Input: part model. Units: mm. Frame: model coordinates. Face numbers are marked on the shaded views. A direction names the side the tool comes from. Give positions to 0.01 mm unless a question says otherwise; leave off trailing zeros. Loops run counter-clockwise (first coordinate to the right, second up) from the corner with the lowest first, then second, coordinate; pieces in that order, holes last. Notation, with made-up numbers: (-17.75, 8.5) -> (-9.75, 8.5) arc R28 ccw to (-9.75, 29.5) -> close; hole circle Ø11 at (3, -28). An arc over 180 degrees is marked (long way). One line per question, with ' | ' between items.
from build123d import *

# Parameters (mm, degrees)
SKETCH1_W           = 120
SKETCH1_H           = 70
BOSS_EXTRUDE1_DEPTH = 10
SKETCH1_3_W         = 20
SKETCH1_3_H         = 70
SKETCH1_3_H_2       = 5.314701235
BOSS_EXTRUDE2_DEPTH = 220
BOSS_EXTRUDE3_START = -20
SKETCH2_W           = 10
SKETCH2_H           = 40
SKETCH2_H_2         = 74.770020504
BOSS_EXTRUDE3_DEPTH = 15
SKETCH3_W           = 59.726354491
SKETCH3_H           = 81.227842107
CUT_EXTRUDE1_DEPTH  = 60
CUT_EXTRUDE2_REACH  = 255.922
CUT_EXTRUDE3_REACH  = 255.922
SKETCH6_W           = 10
SKETCH6_H           = 30
BOSS_EXTRUDE4_DEPTH = 15
CUT_EXTRUDE4_REACH  = 256.324
CUT_EXTRUDE5_REACH  = 256.324


with BuildPart() as part:
    # Sketch1 → Boss-Extrude1 (new body)
    with BuildSketch(Plane(origin=(0, 0, 0), x_dir=(1, 0, 0), z_dir=(0, 1, 0))):
        Rectangle(SKETCH1_W, SKETCH1_H)
        with BuildLine():
            Line((-45.469645663, 21.603573917), (-25.469645663, 21.603573917))
            ThreePointArc((-25.469645663, 21.603573917), (-22.969645663, 19.103573917), (-25.469645663, 16.603573917))
            Line((-25.469645663, 16.603573917), (-45.469645663, 16.603573917))
            ThreePointArc((-45.469645663, 16.603573917), (-47.969645663, 19.103573917), (-45.469645663, 21.603573917))
        make_face(mode=Mode.SUBTRACT)
        with BuildLine():
            Line((45.469645663, 21.603573917), (25.469645663, 21.603573917))
            ThreePointArc((25.469645663, 21.603573917), (22.969645663, 19.103573917), (25.469645663, 16.603573917))
            Line((25.469645663, 16.603573917), (45.469645663, 16.603573917))
            ThreePointArc((45.469645663, 16.603573917), (47.969645663, 19.103573917), (45.469645663, 21.603573917))
        make_face(mode=Mode.SUBTRACT)
        with BuildLine():
            Line((45.469645663, -21.603573917), (25.469645663, -21.603573917))
            ThreePointArc((25.469645663, -21.603573917), (22.969645663, -19.103573917), (25.469645663, -16.603573917))
            Line((25.469645663, -16.603573917), (45.469645663, -16.603573917))
            ThreePointArc((45.469645663, -16.603573917), (47.969645663, -19.103573917), (45.469645663, -21.603573917))
        make_face(mode=Mode.SUBTRACT)
        with BuildLine():
            Line((-45.469645663, -21.603573917), (-25.469645663, -21.603573917))
            ThreePointArc((-25.469645663, -21.603573917), (-22.969645663, -19.103573917), (-25.469645663, -16.603573917))
            Line((-25.469645663, -16.603573917), (-45.469645663, -16.603573917))
            ThreePointArc((-45.469645663, -16.603573917), (-47.969645663, -19.103573917), (-45.469645663, -21.603573917))
        make_face(mode=Mode.SUBTRACT)
    extrude(amount=BOSS_EXTRUDE1_DEPTH)

    # Sketch1<3> → Boss-Extrude2 (add)
    with BuildSketch(Plane(origin=(0, 0, 0), x_dir=(1, 0, 0), z_dir=(0, 1, 0))):
        Rectangle(SKETCH1_3_W, SKETCH1_3_H)
        with Locations((0, 37.657350618)):
            Rectangle(SKETCH1_3_W, SKETCH1_3_H_2)
        with Locations((0, -37.657350618)):
            Rectangle(SKETCH1_3_W, SKETCH1_3_H_2)
    extrude(amount=BOSS_EXTRUDE2_DEPTH)

    # Sketch2 → Boss-Extrude3 (add)
    with BuildSketch(Plane(origin=(10, 0, 0), x_dir=(0, 0, -1), z_dir=(1, 0, 0)).offset(BOSS_EXTRUDE3_START)):
        with Locations((-35, 196.268517414)):
            Rectangle(SKETCH2_W, SKETCH2_H)
        with Locations((35, 195.908265462)):
            Rectangle(SKETCH2_W, SKETCH2_H_2)
    extrude(amount=-BOSS_EXTRUDE3_DEPTH)

    # Sketch3 → Cut-Extrude1 (cut)
    with BuildSketch(Plane(origin=(10, 0, 0), x_dir=(0, 0, -1), z_dir=(1, 0, 0))):
        with Locations((0.081735862, 105.141319111)):
            Rectangle(SKETCH3_W, SKETCH3_H)
    extrude(amount=-CUT_EXTRUDE1_DEPTH, mode=Mode.SUBTRACT)

    # Sketch4 → Cut-Extrude2 (cut, up to next)
    with BuildSketch(Plane.XY.offset(40), mode=Mode.PRIVATE) as cut_extrude2_sk1:
        with BuildLine():
            Line((-14.5, 205.983659563), (-14.5, 190.983659563))
            ThreePointArc((-14.5, 190.983659563), (-17, 188.483659563), (-19.5, 190.983659563))
            Line((-19.5, 190.983659563), (-19.5, 205.983659563))
            ThreePointArc((-19.5, 205.983659563), (-17, 208.483659563), (-14.5, 205.983659563))
        make_face()
    cut_extrude2_tool1 = extrude(cut_extrude2_sk1.sketch, amount=-CUT_EXTRUDE2_REACH, mode=Mode.PRIVATE) & part.part
    add(cut_extrude2_tool1.solids().sort_by_distance((-17, 198.48366, 40))[0], mode=Mode.SUBTRACT)

    # Sketch5 → Cut-Extrude3 (cut, up to next)
    with BuildSketch(Plane(origin=(0, 0, -40), x_dir=(-1, 0, 0), z_dir=(0, 0, -1)), mode=Mode.PRIVATE) as cut_extrude3_sk1:
        with BuildLine():
            Line((19.5, 222.819701207), (19.5, 207.819701207))
            ThreePointArc((19.5, 207.819701207), (17, 205.319701207), (14.5, 207.819701207))
            Line((14.5, 207.819701207), (14.5, 222.819701207))
            ThreePointArc((14.5, 222.819701207), (17, 225.319701207), (19.5, 222.819701207))
        make_face()
    cut_extrude3_tool1 = extrude(cut_extrude3_sk1.sketch, amount=-CUT_EXTRUDE3_REACH, mode=Mode.PRIVATE) & part.part
    # Sketch5 → Cut-Extrude3 (cut, up to next)
    with BuildSketch(Plane(origin=(0, 0, -40), x_dir=(-1, 0, 0), z_dir=(0, 0, -1)), mode=Mode.PRIVATE) as cut_extrude3_sk2:
        with BuildLine():
            Line((19.5, 183.206485392), (19.5, 168.206485392))
            ThreePointArc((19.5, 168.206485392), (17, 165.706485392), (14.5, 168.206485392))
            Line((14.5, 168.206485392), (14.5, 183.206485392))
            ThreePointArc((14.5, 183.206485392), (17, 185.706485392), (19.5, 183.206485392))
        make_face()
    cut_extrude3_tool2 = extrude(cut_extrude3_sk2.sketch, amount=-CUT_EXTRUDE3_REACH, mode=Mode.PRIVATE) & part.part
    add(cut_extrude3_tool1.solids().sort_by_distance((-17, 215.319701, -40))[0], mode=Mode.SUBTRACT)
    add(cut_extrude3_tool2.solids().sort_by_distance((-17, 175.706485, -40))[0], mode=Mode.SUBTRACT)

    # Sketch6 → Boss-Extrude4 (add)
    with BuildSketch(Plane(origin=(10, 0, 0), x_dir=(0, 0, -1), z_dir=(1, 0, 0))):
        with Locations((-35.763941906, 195.796360994)):
            Rectangle(SKETCH6_W, SKETCH6_H)
        with Locations((35.812510383, 213.029875947)):
            Rectangle(SKETCH6_W, SKETCH6_H)
    extrude(amount=BOSS_EXTRUDE4_DEPTH)

    # Sketch7 → Cut-Extrude4 (cut, up to next)
    with BuildSketch(Plane.XY.offset(40.763941906), mode=Mode.PRIVATE) as cut_extrude4_sk1:
        with BuildLine():
            Line((19.5, 203.624140304), (19.5, 188.624140304))
            ThreePointArc((19.5, 188.624140304), (17, 186.124140304), (14.5, 188.624140304))
            Line((14.5, 188.624140304), (14.5, 203.624140304))
            ThreePointArc((14.5, 203.624140304), (17, 206.124140304), (19.5, 203.624140304))
        make_face()
    cut_extrude4_tool1 = extrude(cut_extrude4_sk1.sketch, amount=-CUT_EXTRUDE4_REACH, mode=Mode.PRIVATE) & part.part
    add(cut_extrude4_tool1.solids().sort_by_distance((17, 196.12414, 40.763942))[0], mode=Mode.SUBTRACT)

    # Sketch8 → Cut-Extrude5 (cut, up to next)
    with BuildSketch(Plane(origin=(0, 0, -40.812510383), x_dir=(-1, 0, 0), z_dir=(0, 0, -1)), mode=Mode.PRIVATE) as cut_extrude5_sk1:
        with BuildLine():
            Line((-14.5, 220.7806332), (-14.5, 205.7806332))
            ThreePointArc((-14.5, 205.7806332), (-17, 203.2806332), (-19.5, 205.7806332))
            Line((-19.5, 205.7806332), (-19.5, 220.7806332))
            ThreePointArc((-19.5, 220.7806332), (-17, 223.2806332), (-14.5, 220.7806332))
        make_face()
    cut_extrude5_tool1 = extrude(cut_extrude5_sk1.sketch, amount=-CUT_EXTRUDE5_REACH, mode=Mode.PRIVATE) & part.part
    add(cut_extrude5_tool1.solids().sort_by_distance((17, 213.280633, -40.81251))[0], mode=Mode.SUBTRACT)


solid = part.part
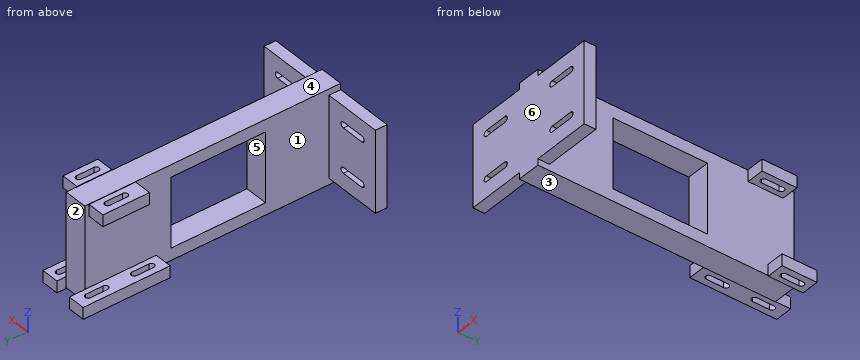
1. Section query A-A (x = 17). Output: boundary loops of the cut face in (y, z).
Determined:
outline: (0, -35) -> (10, -35) -> (10, 35) -> (0, 35) -> close; (180.8, 30.76) -> (186.12, 30.76) -> (186.12, 40.76) -> (180.8, 40.76) -> close; (198.03, -40.81) -> (203.28, -40.81) -> (203.28, -30.81) -> (198.03, -30.81) -> close; (206.12, 30.76) -> (210.8, 30.76) -> (210.8, 40.76) -> (206.12, 40.76) -> close; (223.28, -40.81) -> (228.03, -40.81) -> (228.03, -30.81) -> (223.28, -30.81) -> close
2. Pin query (flat end, axial travel): P1, Ø0.5, axis at y = 203, z = 40.5, coming from the -X side; P2, Ø11, axis at x = -32.5, y = 6.5, coming from the +Z side; P3, Ø5, axis at y = 173, z = -37.5, coming from the +X side. Return the tip coordinate at first contact, or that it passes through.
Determined:
P1: stops at x = -10 | P2: stops at z = 35 | P3: stops at x = 10
3. Pull-direction query (Z, two-part tool) for the marked faces 1, 2 and 3; classes: pulls with the +Z half, pulls with the -Z half, needs draft (parallel to the pull), parting line crosses it, or undercut.
Determined:
face 1: undercut | face 2: needs draft | face 3: pulls with the -Z half
4. Section query B-B (x = -38). Output: boundary loops of the cut face in (y, z).
Determined:
outline: (0, -35) -> (10, -35) -> (10, -21.6) -> (0, -21.6) -> close; (0, -16.6) -> (10, -16.6) -> (10, 16.6) -> (0, 16.6) -> close; (0, 21.6) -> (10, 21.6) -> (10, 35) -> (0, 35) -> close
5. Section query C-C (y = 139.5). Output: boundary loops of the cut face in (x, z).
Determined:
outline: (-10, -40.31) -> (10, -40.31) -> (10, -29.94) -> (-10, -29.94) -> close; (-10, 29.78) -> (10, 29.78) -> (10, 40.31) -> (-10, 40.31) -> close
6. Reachability of the marked faces 4, 5 and 6 from +Z, -Z, +X, -X, +Y, -Y: full face, straight path, thin tool, end or side. Return the list, or none.
Determined:
face 4: +Z, -X, +Y, -Y | face 5: +X, -X | face 6: +Z, -Z, +X, -X, -Y
7. Section query D-D (x = -17). Output: boundary loops of the cut face in (y, z).
Determined:
outline: (0, -35) -> (10, -35) -> (10, 35) -> (0, 35) -> close; (158.52, -40) -> (165.71, -40) -> (165.71, -30) -> (158.52, -30) -> close; (176.27, 30) -> (188.48, 30) -> (188.48, 40) -> (176.27, 40) -> close; (185.71, -40) -> (205.32, -40) -> (205.32, -30) -> (185.71, -30) -> close; (208.48, 30) -> (216.27, 30) -> (216.27, 40) -> (208.48, 40) -> close; (225.32, -40) -> (233.29, -40) -> (233.29, -30) -> (225.32, -30) -> close
8. Ray query, line 1 along Y through (x, z) = (-2, -0.5); line 2 along Z through (x, y) = (3, 125); line 3 along Y through (x, z) = (29, -4). Return the intervals inside material, ascending. Write a range as from..to.
Determined:
line 1: y = 0..64.53, 145.76..220 | line 2: z = -40.31..-29.94, 29.78..40.31 | line 3: y = 0..10
